from build123d import *

# Parameters (mm, degrees)
CROQUIS1_R              = 1.5
CROQUIS1_W              = 23
CROQUIS1_H              = 10.5
CROQUIS1_W_2            = 12
CROQUIS1_H_2            = 20.5
CROQUIS1_W_3            = 8
CROQUIS1_H_3            = 24
CROQUIS1_W_4            = 105
CROQUIS1_H_4            = 35
SALIENTE_EXTRUIR1_DEPTH = 1


with BuildPart() as part:
    # Croquis1 → Saliente-Extruir1 (new body)
    with BuildSketch(Plane.XY):
        with BuildLine():
            Line((-1537.163110479, -136.766453489), (-1516.853146696, -125.6542904))
            ThreePointArc((-1516.853146696, -125.6542904), (-1484.11625712, -138.920059749), (-1457.482039397, -162.121417938))
            Line((-1457.482039397, -162.121417938), (-1445.993940748, -162.121417938))
            Line((-1445.993940748, -162.121417938), (-1445.762202271, -162.121417938))
            ThreePointArc((-1445.762202271, -162.121417938), (-1455.297709344, -223.734904974), (-1497.428135695, -269.693308507))
            Line((-1497.428135695, -269.693308507), (-1552.200391445, -269.693308507))
            Line((-1552.200391445, -269.693308507), (-1606.972647196, -269.693308507))
            ThreePointArc((-1606.972647196, -269.693308507), (-1649.103073546, -223.734904974), (-1658.638580619, -162.121417938))
            Line((-1658.638580619, -162.121417938), (-1646.918743493, -162.121417938))
            ThreePointArc((-1646.918743493, -162.121417938), (-1620.284525771, -138.920059749), (-1587.547636195, -125.6542904))
            Line((-1587.547636195, -125.6542904), (-1567.237672411, -136.766453489))
            ThreePointArc((-1567.237672411, -136.766453489), (-1566.281329143, -132.459607123), (-1564.119167026, -128.614015745))
            Line((-1564.119167026, -128.614015745), (-1566.175134815, -121.889248119))
            Line((-1566.175134815, -121.889248119), (-1559.719031928, -126.933308507))
            Line((-1559.719031928, -126.933308507), (-1544.681750962, -126.933308507))
            Line((-1544.681750962, -126.933308507), (-1538.225648075, -121.889248119))
            Line((-1538.225648075, -121.889248119), (-1540.281615865, -128.614015745))
            ThreePointArc((-1540.281615865, -128.614015745), (-1538.119453748, -132.459607123), (-1537.163110479, -136.766453489))
        make_face()
        with Locations((-1523.716235661, -264.175855838)):
            Circle(CROQUIS1_R, mode=Mode.SUBTRACT)
        with Locations((-1644.551864676, -185.675855838)):
            Circle(CROQUIS1_R, mode=Mode.SUBTRACT)
        with Locations((-1541.502776276, -167.322485879)):
            Circle(CROQUIS1_R, mode=Mode.SUBTRACT)
        with Locations((-1552.400156362, -167.322485879)):
            Circle(CROQUIS1_R, mode=Mode.SUBTRACT)
        with Locations((-1563.201766149, -167.322485879)):
            Circle(CROQUIS1_R, mode=Mode.SUBTRACT)
        with Locations((-1552.400156362, -161.472485879)):
            Circle(CROQUIS1_R, mode=Mode.SUBTRACT)
        with Locations((-1460.786663592, -185.675855838)):
            Circle(CROQUIS1_R, mode=Mode.SUBTRACT)
        with Locations((-1461.847779246, -163.902354835)):
            Circle(CROQUIS1_R, mode=Mode.SUBTRACT)
        with Locations((-1643.220327484, -164.014915474)):
            Circle(CROQUIS1_R, mode=Mode.SUBTRACT)
        with Locations((-1563.201766149, -161.472485879)):
            Circle(CROQUIS1_R, mode=Mode.SUBTRACT)
        with Locations((-1541.502776276, -161.472485879)):
            Circle(CROQUIS1_R, mode=Mode.SUBTRACT)
        with Locations((-1581.083835661, -264.175855838)):
            Circle(CROQUIS1_R, mode=Mode.SUBTRACT)
        with Locations((-1637.158149658, -167.514915474)):
            Circle(CROQUIS1_R, mode=Mode.SUBTRACT)
        with Locations((-1467.909957073, -167.402354835)):
            Circle(CROQUIS1_R, mode=Mode.SUBTRACT)
        with Locations((-1623.732006953, -186.485491114)):
            Circle(CROQUIS1_R, mode=Mode.SUBTRACT)
        with Locations((-1481.067822966, -186.485491114)):
            Circle(CROQUIS1_R, mode=Mode.SUBTRACT)
        with BuildLine():
            Line((-1550.123752332, -261.693308507), (-1506.829937403, -261.693308507))
            ThreePointArc((-1506.829937403, -261.693308507), (-1474.837098768, -233.882364295), (-1457.957337533, -194.997097128))
            ThreePointArc((-1457.957337533, -194.997097128), (-1475.380705089, -191.41817703), (-1493.091376833, -193.065754767))
            Line((-1493.091376833, -193.065754767), (-1501.186287871, -220.101341452))
            Line((-1501.186287871, -220.101341452), (-1525.911955882, -214.031108862))
            Line((-1525.911955882, -214.031108862), (-1550.123752332, -258.096464053))
            Line((-1550.123752332, -258.096464053), (-1550.123752332, -261.693308507))
        make_face(mode=Mode.SUBTRACT)
        with BuildLine():
            Line((-1578.488827009, -214.031108862), (-1554.277030559, -258.096464053))
            Line((-1554.277030559, -258.096464053), (-1554.277030559, -261.693308507))
            Line((-1554.277030559, -261.693308507), (-1597.570845488, -261.693308507))
            ThreePointArc((-1597.570845488, -261.693308507), (-1629.563684123, -233.882364295), (-1646.443445358, -194.997097128))
            ThreePointArc((-1646.443445358, -194.997097128), (-1629.020077802, -191.41817703), (-1611.309406057, -193.065754767))
            Line((-1611.309406057, -193.065754767), (-1603.21449502, -220.101341452))
            Line((-1603.21449502, -220.101341452), (-1578.488827009, -214.031108862))
        make_face(mode=Mode.SUBTRACT)
        with Locations((-1552.400156362, -229.832455111)):
            Rectangle(CROQUIS1_W, CROQUIS1_H, mode=Mode.SUBTRACT)
        with Locations((-1489.400156362, -166.947886235)):
            Rectangle(CROQUIS1_W_2, CROQUIS1_H_2, mode=Mode.SUBTRACT)
        with Locations((-1615.400156362, -166.947886235)):
            Rectangle(CROQUIS1_W_2, CROQUIS1_H_2, mode=Mode.SUBTRACT)
        with Locations((-1552.200391445, -143.53903119)):
            Rectangle(CROQUIS1_W_3, CROQUIS1_H_3, mode=Mode.SUBTRACT)
        with Locations((-1552.400156362, -187.822466505)):
            Rectangle(CROQUIS1_W_4, CROQUIS1_H_4, mode=Mode.SUBTRACT)
    extrude(amount=SALIENTE_EXTRUIR1_DEPTH)


solid = part.part
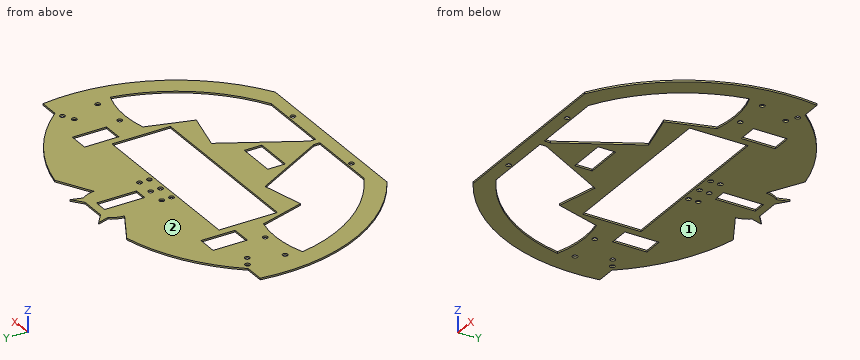
Read the model definition and answer for the solid it produces. Units are mm, in the model's axes. Face numbers are marked on the shaded views. Coordinates: 2 decimals unless noted, no trailing zeros. Order: outer loops, then holes, each group sorted by start corner. A loop starts at its lowest first (then second) coordinate and runs counter-clockwise, first axis right, second up. Notation, with made-up numbers: (60.25, -31.75) -> (66.25, -31.75) arc R26 ccw to (66.25, -13.75) -> close; hole circle Ø2 at (52, -29.75). An arc over 180 degrees is marked (long way). Answer as a JSON object with one key per item and string values.
1) The mould has two halves that part along Z. Classify the marked faces 1 and 2: released by +Z, released by -Z, zero draft, split by the parting line, or undercut.
Model answer:
{"face 1": "released by -Z", "face 2": "released by +Z"}
2) Consider line 1 along X through (y, z) = (-242, 0.1); line 2 along Y through (x, z) = (-1483.5, 0.1); line 3 along Y through (x, z) = (-1468, 0.55). Determine where each line is inside the solid, lowest interval first. Write a range as from..to.
Model answer:
{"line 1": "x = -1637.97..-1622.9, -1563.12..-1541.28, -1481.5..-1466.43", "line 2": "y = -259.88..-244.12, -191.52..-177.2, -156.7..-139.3", "line 3": "y = -244.03..-223.12, -192.28..-168.9, -165.91..-151.05"}
3) A cutting plane is placed at C-C, the plane y = -141. Determine the outline of the cut face in (x, z).
Model answer:
{"outline": "(-1623.54, 0) -> (-1556.2, 0) -> (-1556.2, 1) -> (-1623.54, 1) -> close; (-1548.2, 0) -> (-1480.86, 0) -> (-1480.86, 1) -> (-1548.2, 1) -> close"}
4) A cutting plane is placed at B-B, the plane x = -1629. Determine the outline of the cut face in (y, z), plus the area to 3 significant figures.
Model answer:
{"outline": "(-252.41, 0) -> (-234.64, 0) -> (-234.64, 1) -> (-252.41, 1) -> close; (-191.42, 0) -> (-144.88, 0) -> (-144.88, 1) -> (-191.42, 1) -> close", "area": "64.3 mm²"}
5) A cutting plane is placed at D-D, the plane z = 0.25. State how many separate pieces and enclosed holes the cut face has, plus the area to 3 significant figures.
Model answer:
{"separate pieces": "1", "enclosed holes": "23", "area": "13,600 mm²"}
6) A cutting plane is placed at A-A, the plane y = -198. Determine the outline of the cut face in (x, z), plus the area to 3 significant figures.
Model answer:
{"outline": "(-1657.67, 0) -> (-1645.83, 0) -> (-1645.83, 1) -> (-1657.67, 1) -> close; (-1609.83, 0) -> (-1604.9, 0) -> (-1604.9, 1) -> (-1609.83, 1) -> close; (-1499.9, 0) -> (-1494.57, 0) -> (-1494.57, 1) -> (-1499.9, 1) -> close; (-1458.57, 0) -> (-1446.73, 0) -> (-1446.73, 1) -> (-1458.57, 1) -> close", "area": "33.9 mm²"}
7) Each of these flat-tipped pins is pushed along its axis until it touches: pin 1 (4 mm diameter, centred on x = -1460.79, y = -185.68, fed in from +Z); pin 2 (0.5 mm diameter, centred on x = -1451, z = 0.5, fed in from +Y); pin 3 (2.5 mm diameter, centred on x = -1523.72, y = -264.18, fed in from +Z); pin 4 (0.5 mm diameter, centred on y = -171, z = 0.5, fed in from -X). Where does it stop, or does it pass through?
Model answer:
{"pin 1": "stops at z = 1", "pin 2": "stops at y = -162.12", "pin 3": "passes through", "pin 4": "stops at x = -1659.54"}
